For this review, use the dimensioned drawing (mm, ordinates from the lowest corner) and the shaded views. Coordinates: 2 decimals unless noted, no trailing zeros. Loops run counter-clockwise (first coordinate to the right, second up) from the corner with the lowest first, then second, coordinate; pieces in that order, holes last. Notation, with made-up numbers: M 71.5,34.25 L 85.5,34.25 A34 ccw 85.5,68.25 Z; hole C 42,32.5 d1. An arc over 180 degrees is marked long. Write item = value, one per line. Start each with the question number.
Q1. We need section A-A on x = 21. Give the boundary of the cut face in (y, z), and give its area (3 significant figures).
Q2. Clearance check with flat-ended pins moving along their axes: pin 1 Ø3 at (x, z) = (19, 22.5) entering from -Y; pin 2 Ø3 at (x, z) = (5.5, 5.5) entering from -Y; pin 3 Ø3.5 at (x, z) = (36.5, 36.5) entering from -Y. State where each tip first meets the part, or that it passes through.
Q3. We need section D-D on y = 7. Give the boundary of the cut face in (x, z), and give its area (3 significant figures).
Q4. Mouldability with a two-part tool opening along Z and no side actions: class the marked faces 1, 2, 3 and 4 as released by +Z, released by -Z, zero draft, split by the parting line, or undercut.
Q5. Wall thickness on probe 1 along Z at (x, y) = (5.5, 3.5); probe 2 along Z at (x, y) = (21, 1.6): over which ranges is each line inside the solid? List them lowest first.
Q6. We need section C-C on x = 5.5. Give the boundary of the cut face in (y, z).
Q7. We need section B-B on z = 36.5. Give the boundary of the cut face in (x, y).
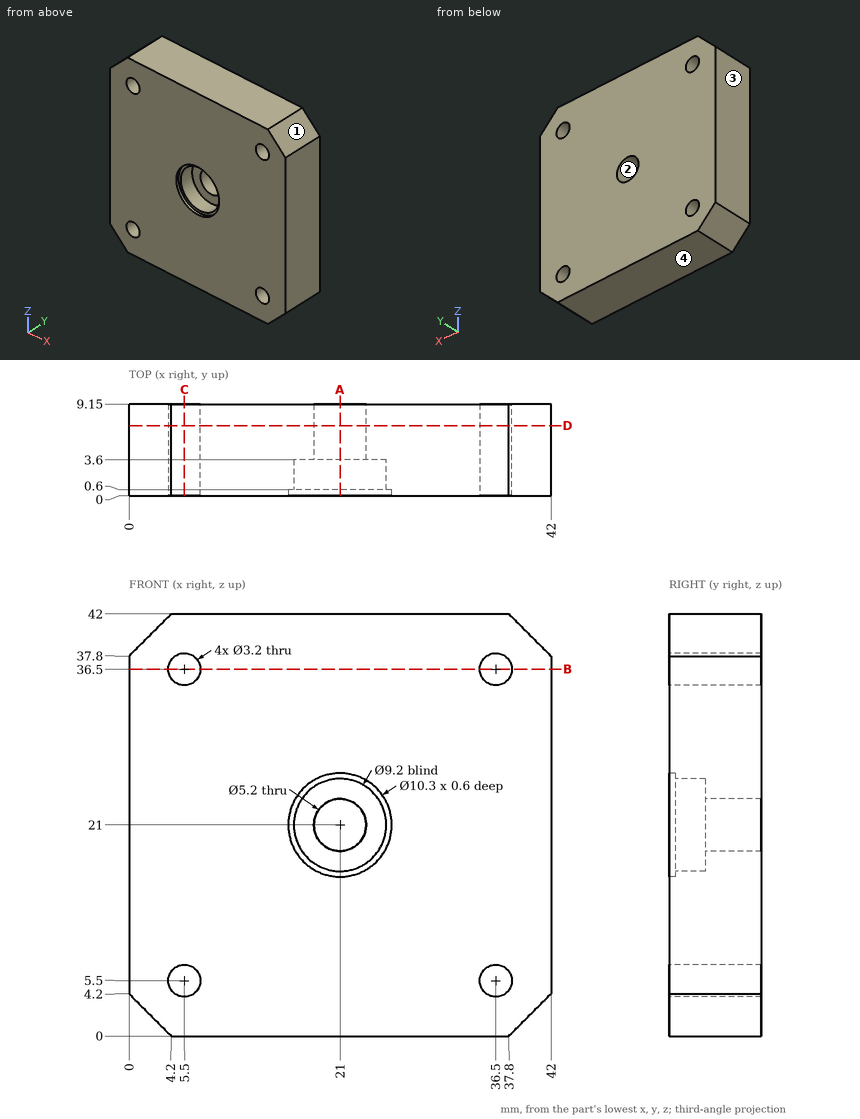
Returned:
q1.outline = M 0,0 L 9.15,0 L 9.15,18.4 L 3.6,18.4 L 3.6,16.4 L 0.6,16.4 L 0.6,15.85 L 0,15.85 Z; M 0,26.15 L 0.6,26.15 L 0.6,25.6 L 3.6,25.6 L 3.6,23.6 L 9.15,23.6 L 9.15,42 L 0,42 Z
q1.area = 322 mm^2
q2.pin_1 = 3.6
q2.pin_2 = through
q2.pin_3 = 0
q3.outline = M 0,4.2 L 4.2,0 L 37.8,0 L 42,4.2 L 42,37.8 L 37.8,42 L 4.2,42 L 0,37.8 Z; hole C 5.5,5.5 d3.2; hole C 5.5,36.5 d3.2; hole C 21,21 d5.2; hole C 36.5,5.5 d3.2; hole C 36.5,36.5 d3.2
q3.area = 1,680 mm^2
q4.face_1 = released by +Z
q4.face_2 = undercut
q4.face_3 = zero draft
q4.face_4 = released by -Z
q5.probe_1 = 0 to 3.9, 7.1 to 34.9, 38.1 to 42
q5.probe_2 = 0 to 16.4, 25.6 to 42
q6.outline = M 0,0 L 9.15,0 L 9.15,3.9 L 0,3.9 Z; M 0,7.1 L 9.15,7.1 L 9.15,34.9 L 0,34.9 Z; M 0,38.1 L 9.15,38.1 L 9.15,42 L 0,42 Z
q7.outline = M 0,0 L 3.9,0 L 3.9,9.15 L 0,9.15 Z; M 7.1,0 L 34.9,0 L 34.9,9.15 L 7.1,9.15 Z; M 38.1,0 L 42,0 L 42,9.15 L 38.1,9.15 Z
